```python
from build123d import *

# Parameters (mm, degrees)
SKETCH_1_W      = 80
SKETCH_1_H      = 50
EXTRUDE_1_DEPTH = 20
SKETCH_2_R      = 2.5
EXTRUDE_2_DEPTH = 1.5


with BuildPart() as part:
    # 草图1 → 凸台-拉伸1 (new body)
    with BuildSketch(Plane.XY):
        Rectangle(SKETCH_1_W, SKETCH_1_H)
    extrude(amount=EXTRUDE_1_DEPTH)

    # 草图2 → 凸台-拉伸2 (add, symmetric)
    with BuildSketch(Plane(origin=(0, 0, 0), x_dir=(1, 0, 0), z_dir=(0, 1, 0))):
        with BuildLine():
            Line((-15, 0), (15, 0))
            ThreePointArc((15, 0), (0, 15), (-15, 0))
        make_face()
        with Locations(Location((0, 8, 0), (0, 0, 270))):
            Circle(SKETCH_2_R, mode=Mode.SUBTRACT)
    extrude(amount=EXTRUDE_2_DEPTH, both=True)


solid = part.part
```
Source: CAD feature listing. Evaluate the final solid. Frame: model axes, mm. A direction names the side the tool comes from. Coordinates: 2 decimals unless noted, no trailing zeros. Order: outer loops, then holes, each group sorted by start corner. A loop starts at its lowest first (then second) coordinate and runs counter-clockwise, first axis right, second up. Notation, with made-up numbers: (-19.75, -4.75) - (14.25, -4.75) arc R19 ccw to (14.25, 24.25) - close; hole circle Ø3 at (-7.5, 44). An arc over 180 degrees is marked (long way). One line per item, written item: value.
1) Cut plane C-C on y = -21. Output: boundary loops of the cut face in (x, z), plus the area to 3 significant figures.
Computed values:
outline: (-40, 0) - (40, 0) - (40, 20) - (-40, 20) - close
area: 1,600 mm^2
2) Cut plane D-D on x = 19. Output: boundary loops of the cut face in (y, z), plus the area to 3 significant figures.
Computed values:
outline: (-25, 0) - (25, 0) - (25, 20) - (-25, 20) - close
area: 1,000 mm^2
3) Contact query for flat-ended pins moving along their axis: pin 1 (7.5 mm diameter, centred on x = 6, z = -8, fed in from +Y); pin 2 (15 mm diameter, centred on x = 8, y = -6, fed in from -Z); pin 3 (4 mm diameter, centred on x = 7.5, y = -15, fed in from -Z). Output: stop coordinate, or through.
Computed values:
pin 1: stops at y = 1.5
pin 2: stops at z = -14.87
pin 3: stops at z = 0
4) Ray query, line 1 (Z direction, x = 11.5, y = -11.5); line 2 (X direction, y = 0, z = -8); line 3 (X direction, y = 0, z = -10). Return the intervals inside material, ascending. Write a range as [from, to].
Computed values:
line 1: z = [0, 20]
line 2: x = [-12.69, -2.5], [2.5, 12.69]
line 3: x = [-11.18, -1.5], [1.5, 11.18]
5) Reachability of faces 5 (the face through (-1, 25, 10)), 6 (the face through (0, -1.5, -4)) from +Z, -Z, +X, -X, +Y, -Y: full face, straight path, thin tool, end or side. Return the list, or none.
Computed values:
face 5: +Z, -Z, +X, -X, +Y
face 6: -Z, +X, -X, -Y
6) Cut plane B-B on z = -8. Output: boundary loops of the cut face in (x, y), plus the area to 3 significant figures.
Computed values:
outline: (-12.69, -1.5) - (-2.5, -1.5) - (-2.5, 1.5) - (-12.69, 1.5) - close; (2.5, -1.5) - (12.69, -1.5) - (12.69, 1.5) - (2.5, 1.5) - close
area: 61.1 mm^2
7) Mould query, pull axis Z, two halves, no side actions, for faces 1 (the face through (0.1, 0, -10.5)), 2 (the face through (0, 1.5, -4)), 3 (the face through (-1, 0, 20)), 4 (the face through (-1, 6, 0)). Classes: released by +Z, released by -Z, zero draft, split by the parting line, or undercut.
Computed values:
face 1: undercut
face 2: zero draft
face 3: released by +Z
face 4: released by -Z
8) Cut plane A-A on x = 0. Output: boundary loops of the cut face in (y, z), plus the area to 3 significant figures.
Computed values:
outline: (-25, 0) - (-1.5, 0) - (-1.5, -5.5) - (1.5, -5.5) - (1.5, 0) - (25, 0) - (25, 20) - (-25, 20) - close; (-1.5, -15) - (1.5, -15) - (1.5, -10.5) - (-1.5, -10.5) - close
area: 1,030 mm^2
